Input: part model. Units: mm. Frame: model coordinates. A direction names the side the tool comes from. Coordinates: 2 decimals unless noted, no trailing zeros.
1) Draft query along Y for faces 1 (the cylindrical face through (9.569, 0.279, -107.956)), 2 (the flat face through (6, -1, 127)), 3 (the flat face through (6, 76.2, 2)), 4 (the flat face through (6.35, 0, -114)). Return one class per face: pulls with the +Y half, pulls with the -Y half, needs draft (parallel to the pull), parting line crosses it, or undercut.
2) Set-up query: faces 5 (the cylindrical face through (5.55, -69.76, 117.4)), 6 (the flat face through (10, -8.635, 27)), 7 (the flat face through (12.7, 1, -26)). Return all of +Z, -Z, +X, -X, +Y, -Y with unobstructed straight access to the full face (end or side cutting, diameter ignored); none if empty.
3) Line query: L1, parallel to X at y = -71, z = 114.3; L2, parallel to Z at x = 10.5, y = 5; L3, parallel to Y at x = 8.75, z = 9. Output: solid intervals per line, ascending.
4) Pin query (flat end, axial travel): pin 1 Ø10 at (y, z) = (0, -114.3) entering from +X. Return the tip coordinate at first contact, or that it passes through.
from build123d import *

# Parameters (mm, degrees)
SKETCH1_W                       = 254
SKETCH1_H                       = 152.4
BOSS_EXTRUDE1_DEPTH             = 12.7
SKETCH3_R                       = 6.35
CUT_EXTRUDE2_DEPTH              = 6.35
F_1_4_0_25_DIAMETER_HOLE1_D     = 6.35
F_1_4_0_25_DIAMETER_HOLE1_DEPTH = 12.7
F_1_4_0_25_DIAMETER_HOLE1_TIP   = 1.907732465
CUT_EXTRUDE3_DEPTH              = 6.35
FILLET1_R                       = 7.62


with BuildPart() as part:
    # Sketch1 → Boss-Extrude1 (new body)
    with BuildSketch(Plane(origin=(0, 0, 0), x_dir=(0, 0, -1), z_dir=(1, 0, 0))):
        Rectangle(SKETCH1_W, SKETCH1_H)
    extrude(amount=BOSS_EXTRUDE1_DEPTH)

    # Sketch3 → Cut-Extrude2 (cut)
    with BuildSketch(Plane(origin=(12.7, 0, 0), x_dir=(0, 0, -1), z_dir=(1, 0, 0))):
        with Locations((114.3, 0)):
            Circle(SKETCH3_R)
        with Locations((-114.3, 0)):
            Circle(SKETCH3_R)
    extrude(amount=-CUT_EXTRUDE2_DEPTH, mode=Mode.SUBTRACT)

    # 1/4 (0.25) Diameter Hole1
    with Locations(Plane(origin=(0, -76.2, 0), x_dir=(-1, 0, 0), z_dir=(0, -1, 0))):
        with Locations((-6.236337014, -114.3), (-6.236337014, 0), (-6.236337014, 114.3)):
            Hole(F_1_4_0_25_DIAMETER_HOLE1_D / 2, depth=F_1_4_0_25_DIAMETER_HOLE1_DEPTH)
            with Locations((0, 0, -(F_1_4_0_25_DIAMETER_HOLE1_DEPTH + F_1_4_0_25_DIAMETER_HOLE1_TIP / 2))):  # 118° drill point
                Cone(0, F_1_4_0_25_DIAMETER_HOLE1_D / 2, F_1_4_0_25_DIAMETER_HOLE1_TIP, mode=Mode.SUBTRACT)

    # Sketch7 → Cut-Extrude3 (cut)
    with BuildSketch(Plane(origin=(12.7, 0, 0), x_dir=(0, 0, -1), z_dir=(1, 0, 0))):
        with BuildLine():
            Line((0, 10.032875442), (0, -8.634963037))
            Line((0, -8.634963037), (-17.653050426, -8.634963037))
            ThreePointArc((-17.653050426, -8.634963037), (4.431634546, -19.145584119), (19.651788112, 0))
            ThreePointArc((19.651788112, 0), (5.202001486, 18.950777201), (-16.897756844, 10.032875442))
            Line((-16.897756844, 10.032875442), (0, 10.032875442))
        make_face()
        with BuildLine():
            Line((-17.653050426, -8.634963037), (0, -8.634963037))
            Line((0, -8.634963037), (0, 10.032875442))
            Line((0, 10.032875442), (-16.897756844, 10.032875442))
            ThreePointArc((-16.897756844, 10.032875442), (-19.635723036, 0.79445382), (-17.653050426, -8.634963037))
        make_face()
        with BuildLine():
            Line((-32.324736448, -8.634963037), (-17.653050426, -8.634963037))
            ThreePointArc((-17.653050426, -8.634963037), (-19.635723036, 0.79445382), (-16.897756844, 10.032875442))
            Line((-16.897756844, 10.032875442), (-32.324736448, 10.032875442))
            Line((-32.324736448, 10.032875442), (-32.324736448, -8.634963037))
        make_face()
    extrude(amount=-CUT_EXTRUDE3_DEPTH, mode=Mode.SUBTRACT)

    # Fillet1
    fillet1_edges = [part.edges().sort_by_distance(p)[0] for p in [
        (9.525, 10.032875442, 16.897756844),
        (9.525, -8.634963037, 17.653050426),
    ]]
    fillet(fillet1_edges, radius=FILLET1_R)


solid = part.part
Answer:
1. face 1: undercut
1. face 2: needs draft
1. face 3: pulls with the +Y half
1. face 4: undercut
2. face 5: -Y
2. face 6: +X
2. face 7: +Z, -Z, +X, +Y, -Y
3. L1: x = 0 to 3.06, 9.41 to 12.7
3. L2: z = -127 to -118.21, -110.39 to -19.01, 32.32 to 110.39, 118.21 to 127
3. L3: y = -76.2 to -17.47, 17.47 to 76.2
4. pin 1: stops at x = 6.35
